Work out the finished part from the listing and answer in its coordinate system (mm). Coordinates: 2 decimals unless noted, no trailing zeros. Order: outer loops, then holes, each group sorted by start corner. A loop starts at its lowest first (then second) coordinate and runs counter-clockwise, first axis right, second up. Notation, with made-up numbers: (-9, 80.25) - (47, 80.25) arc R9 ccw to (47, 92.25) - close; hole circle Ø11 at (8, 77.5). An arc over 180 degrees is marked (long way). Answer as a JSON object with one key per item and string values. Group by question number.
1) Each of these flat-tipped pins is pushed along its axis until it touches: P1, Ø1.5, axis at y = 159, z = -2, coming from the +X side; P2, Ø8, axis at x = 1.47, y = 213.86, coming from the +Z side; P3, Ø1.5, axis at y = 165.5, z = -2, coming from the -X side; P4, Ø5, axis at x = 33.78, y = 57.16, coming from the -Z side. Where does it stop, or does it pass through?
2) Find the intervals of material crossed by line 1 along X through (y, z) = (59.5, -1.55); line 2 along X through (y, z) = (172.5, -2); line 3 along X through (y, z) = (83, -0.85), in increasing order.
3) Section A-A (z = -1.35) is taken. Give the vertices of the cut face in (x, y), plus the area to 3 significant figures.
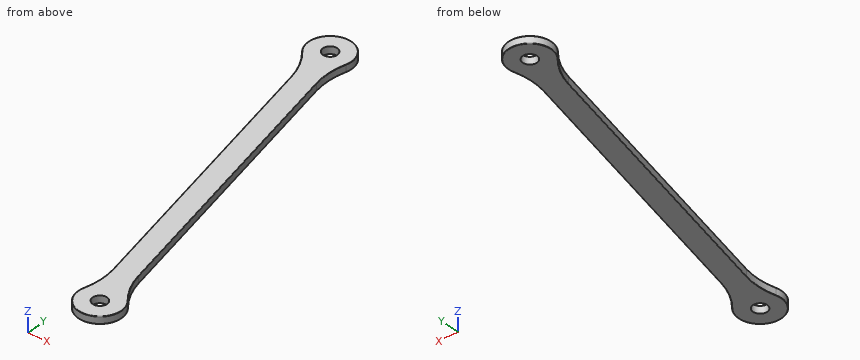
from build123d import *

# Parameters (mm, degrees)
BOSS_EXTRUDE1_DEPTH = 3
FILLET1_R           = 30
FILLET2_R           = 0.15
SKETCH2_R           = 4.65
SKETCH2_R_2         = 3
BOSS_EXTRUDE2_DEPTH = 3


with BuildPart() as part:
    # Sketch1 → Boss-Extrude1 (new body)
    with BuildSketch(Plane.XY):
        with BuildLine():
            ThreePointArc((7.448612374, 207.134028056), (-0.350164285, 222.673500313), (-1.365961708, 205.316534248))
            Line((-1.365961708, 205.316534248), (-2.939957518, 212.950179327))
            ThreePointArc((-2.939957518, 212.950179327), (0.558582619, 218.266213272), (5.874616565, 214.767673135))
            Line((5.874616565, 214.767673135), (7.448612374, 207.134028056))
        make_face()
        with BuildLine():
            Line((29.371043524, 56.246640082), (-2.939957518, 212.950179327))
            ThreePointArc((-2.939957518, 212.950179327), (2.376076428, 209.45163919), (5.874616565, 214.767673135))
            Line((5.874616565, 214.767673135), (38.185617606, 58.064133891))
            ThreePointArc((38.185617606, 58.064133891), (32.869583661, 61.562674028), (29.371043524, 56.246640082))
        make_face()
        with BuildLine():
            ThreePointArc((38.185617606, 58.064133891), (34.687077469, 52.748099945), (29.371043524, 56.246640082))
            Line((29.371043524, 56.246640082), (27.797047714, 63.880285161))
            ThreePointArc((27.797047714, 63.880285161), (35.595824373, 48.340812904), (36.611621797, 65.69777897))
            Line((36.611621797, 65.69777897), (38.185617606, 58.064133891))
        make_face()
    extrude(amount=-BOSS_EXTRUDE1_DEPTH)

    # Fillet1
    fillet1_edges = [part.edges().sort_by_distance(p)[0] for p in [
        (-1.365961708, 205.316534248, -1.5),
        (7.448612374, 207.134028056, -1.5),
        (36.611621797, 65.69777897, -1.5),
        (27.797047714, 63.880285161, -1.5),
    ]]
    fillet(fillet1_edges, radius=FILLET1_R)

    # Fillet2
    fillet2_edges = [part.edges().sort_by_distance(p)[0] for p in [
        (35.595824373, 48.340812904, 0),
        (35.595824373, 48.340812904, -3),
        (22.030117085, 136.415903513, 0),
        (22.030117085, 136.415903513, -3),
        (5.874616565, 214.767673135, -3),
        (13.215543003, 134.598409705, 0),
        (13.215543003, 134.598409705, -3),
        (-0.350164285, 222.673500313, 0),
        (-0.350164285, 222.673500313, -3),
        (36.828265789, 68.99602006, 0),
        (36.828265789, 68.99602006, -3),
        (26.293400844, 66.823816204, 0),
        (26.293400844, 66.823816204, -3),
        (-1.582605701, 202.018293157, 0),
        (34.687077469, 52.748099945, -3),
        (-1.582605701, 202.018293157, -3),
        (8.952259244, 204.190497013, 0),
        (8.952259244, 204.190497013, -3),
        (34.687077469, 52.748099945, 0),
        (5.874616565, 214.767673135, 0),
    ]]
    fillet(fillet2_edges, radius=FILLET2_R)

    # Sketch2 → Boss-Extrude2 (add)
    with BuildSketch(Plane.XY):
        with Locations((1.467329524, 213.858926231)):
            Circle(SKETCH2_R)
        with Locations((1.467329524, 213.858926231)):
            Circle(SKETCH2_R_2, mode=Mode.SUBTRACT)
        with Locations((33.778330565, 57.155386987)):
            Circle(SKETCH2_R)
        with Locations((33.778330565, 57.155386987)):
            Circle(SKETCH2_R_2, mode=Mode.SUBTRACT)
    extrude(amount=-BOSS_EXTRUDE2_DEPTH)


solid = part.part
Report:
{
 "1": {"P1": "stops at x = 17.53", "P2": "stops at z = 0", "P3": "stops at x = 6.69", "P4": "passes through"},
 "2": {"line 1": "x = 25.09 to 31.91, 35.65 to 42.47", "line 2": "x = 5.4 to 14.59", "line 3": "x = 23.85 to 33.04"},
 "3": {"outline": "(-5.48, 208.14) arc R30 cw to (0.73, 195.14) - (25.7, 74.06) arc R30 cw to (25.13, 59.66) arc R9 ccw (long way) to (40.73, 62.87) arc R30 cw to (34.51, 75.88) - (9.55, 196.96) arc R30 cw to (10.11, 211.36) arc R9 ccw (long way) to start; hole circle Ø6 at (1.47, 213.86); hole circle Ø6 at (33.78, 57.16)", "area": "1,770 mm²"}
}
